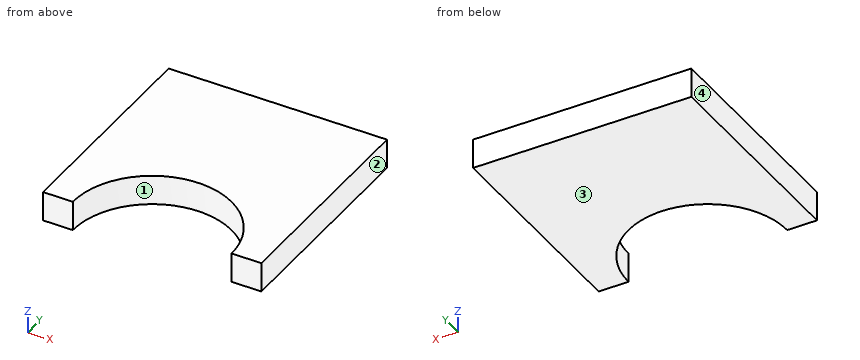
```python
from build123d import *

# Parameters (mm, degrees)
F1_DEPTH = 19.05


with BuildPart() as f1:
    # F0 (on Top) → F1 (new body)
    with BuildSketch(Plane.XY):
        with BuildLine():
            Line((69.849999, -69.709386), (69.849999, 69.990614))
            Line((69.849999, 69.990614), (-69.850001, 69.990614))
            Line((-69.850001, 69.990614), (-69.850001, -69.709386))
            Line((-69.850001, -69.709386), (-50.800001, -69.709386))
            ThreePointArc((-50.800001, -69.709386), (-1e-06, -18.909386), (50.799999, -69.709386))
            Line((50.799999, -69.709386), (69.849999, -69.709386))
        make_face()
    extrude(amount=F1_DEPTH)


solid = f1.part
```
For this review, take the finished solid that the model builds, in its own axes (mm). Face numbers are marked on the shaded views. Coordinates: 2 decimals unless noted, no trailing zeros. Write each loop counter-clockwise with the first axis right and the second up, starting at its lowest first coordinate (ties: lowest second). Pieces come first, ordered by that corner, then holes. Notation, with made-up numbers: (14, 28.25) - (33, 28.25) arc R24 cw to (33, 42.25) - close; hole circle Ø2 at (-35.5, -30.5). An arc over 180 degrees is marked (long way). Answer in a Markdown table with one row per item. Add a question column.
Q1. Draft analysis for pull direction X (two halves, no side actions). For the marked faces 1, 2, 3 and 4, state which applies: +X half, -X half, draft (parallel to the pull), parting line (faces both ways), or undercut.
Q2. We need section B-B, the plane x = 0. State the section outline as (y, z) points, and give its area (3 significant figures).
Q3. For P1, Ø1.5, axis at x = -10.5, z = 13, coming from the -Y side; P2, Ø6, axis at x = 45.5, y = 35.5, coming from the -Z side, all flat-tipped, find the tip position at first contact; note any pin that passes through.
Q4. We need section C-C, the plane x = -48. State the section outline as (y, z) points.
Q5. For probe 1 along X at (y, z) = (-59, 11.5); probe 2 along X at (y, z) = (-40, 11); probe 3 along Y at (x, z) = (-7.5, 5.5), list the stretches that pass through material, from the lowest coordinate up.
Q6. We need section A-A, the plane z = 14.25. State the section outline as (x, y) points.
Answer list:
| question | item | result |
|---|---|---|
| 1 | face 1 | undercut |
| 1 | face 2 | +X half |
| 1 | face 3 | draft |
| 1 | face 4 | -X half |
| 2 | outline | (-18.91, 0) - (69.99, 0) - (69.99, 19.05) - (-18.91, 19.05) - close |
| 2 | area | 1,690 mm2 |
| 3 | P1 | stops at y = -20.17 |
| 3 | P2 | stops at z = 0 |
| 4 | outline | (-53.08, 0) - (69.99, 0) - (69.99, 19.05) - (-53.08, 19.05) - close |
| 5 | probe 1 | x = -69.85 to -49.66, 49.66 to 69.85 |
| 5 | probe 2 | x = -69.85 to -41.21, 41.21 to 69.85 |
| 5 | probe 3 | y = -19.47 to 69.99 |
| 6 | outline | (-69.85, -69.71) - (-50.8, -69.71) arc R50.8 cw to (50.8, -69.71) - (69.85, -69.71) - (69.85, 69.99) - (-69.85, 69.99) - close |
